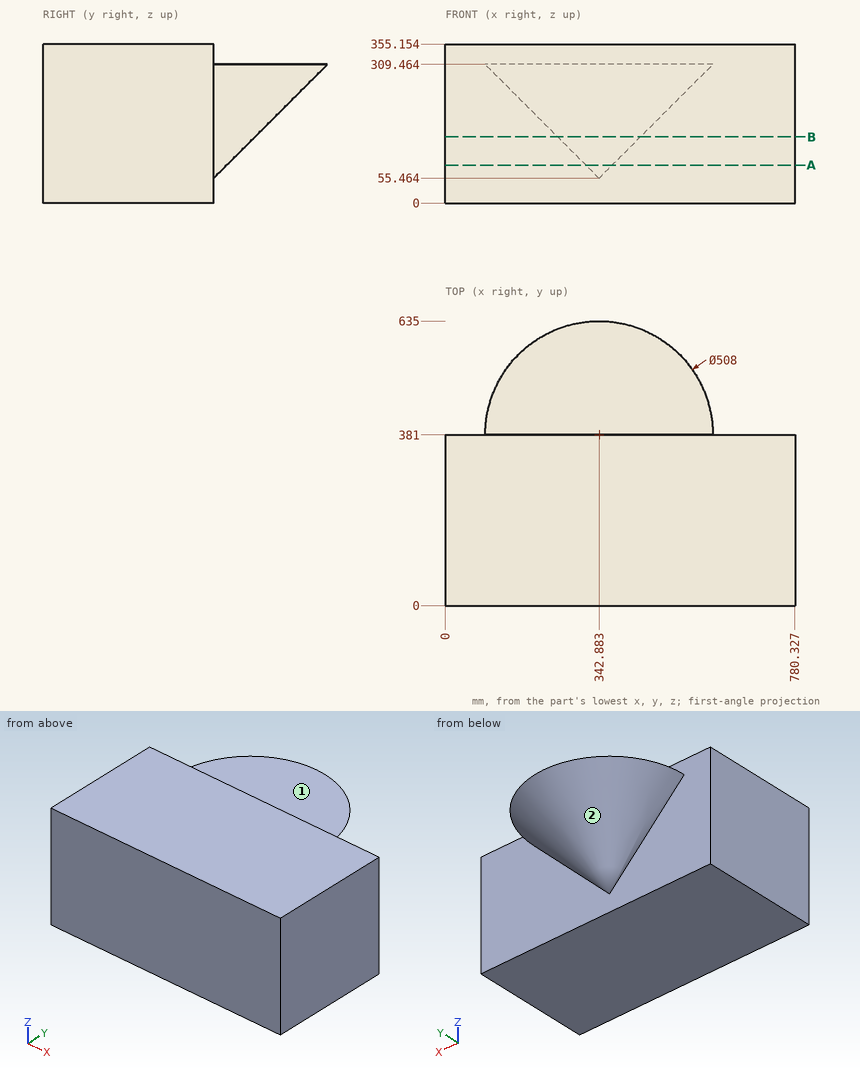
Geometry: see drawing. Coordinates: mm, zero at the bounding-box minimum. A direction names the side the tool comes from. Give positions to 0.01 mm unless a question says otherwise; leave off trailing zeros. Write each loop counter-clockwise with the first axis right and the second up, starting at its lowest first coordinate (ties: lowest second). Pieces come first, ordered by that corner, then holes. Notation, with made-up numbers: (45, 79.5) - (83, 79.5) arc R20 cw to (83, 102.5) - close; hole circle Ø1 at (30, 31.25). An arc over 180 degrees is marked (long way). Return JSON: item names as keys, results as strings. Group by question number.
1) Set-up query: the marked faces 1 and 2. Return all of +Z, -Z, +X, -X, +Y, -Y with unobstructed straight access to the full face (end or side cutting, diameter ignored); none if empty.
2) Section B-B on z = 148. Return the cut outline in (x, y) (1 decimal).
3) Section A-A on z = 84.5. Return the cut outline in (x, y) (1 decimal).
4) Line query: line 1 (Y direction, x = 548, z = 17.5); line 2 (Y direction, x = 379, z = 220.5) (1 decimal); line 3 (Z direction, x = 555.5, y = 407) (1 decimal). Output: solid intervals per line, ascending.
5) First-contact query: P1, Ø12, axis at x = 571, y = 502.5, coming from the +Z side; P2, Ø12, axis at x = 527.5, y = 543, coming from the -Z side; P3, Ø5, axis at x = 181.5, z = 271, coming from the +Y side. Flat tips, straight axial feed; report the tip coordinate or a pass-through.
Filled in:
{
 "1": {"face 1": "+Z, +X, -X, +Y", "face 2": "-Z, +Y"},
 "2": {"outline": "(0, 0) - (780.3, 0) - (780.3, 381) - (435.4, 381) arc R92.5 ccw to (250.3, 381) - (0, 381) - close"},
 "3": {"outline": "(0, 0) - (780.3, 0) - (780.3, 381) - (371.9, 381) arc R29 ccw to (313.8, 381) - (0, 381) - close"},
 "4": {"line 1": "y = 0 to 381", "line 2": "y = 0 to 542", "line 3": "z = 269.7 to 309.5"},
 "5": {"P1": "stops at z = 309.46", "P2": "stops at z = 295.08", "P3": "stops at y = 528.51"}
}
